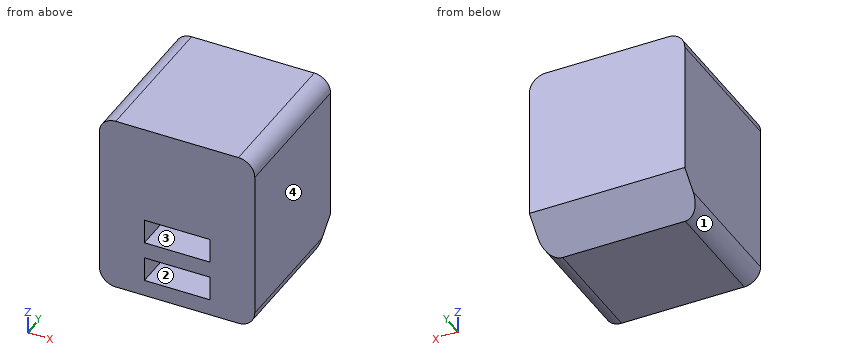
from build123d import *

# Parameters (mm, degrees)
F1_DEPTH = 28.575
F3_DEPTH = 30.1635
F6_W     = 12.7
F6_H     = 4.7625
F7_DEPTH = 12.7


with BuildPart() as f1:
    # F0 (on Front) → F1 (new body)
    with BuildSketch(Plane.XZ):
        with BuildLine():
            ThreePointArc((15.08125, 14.2875), (14.151314, 16.532564), (11.90625, 17.4625))
            Line((11.90625, 17.4625), (-11.90625, 17.4625))
            ThreePointArc((-11.90625, 17.4625), (-14.151314, 16.532564), (-15.08125, 14.2875))
            Line((-15.08125, 14.2875), (-15.08125, -14.2875))
            ThreePointArc((-15.08125, -14.2875), (-14.151314, -16.532564), (-11.90625, -17.4625))
            Line((-11.90625, -17.4625), (11.90625, -17.4625))
            ThreePointArc((11.90625, -17.4625), (14.151314, -16.532564), (15.08125, -14.2875))
            Line((15.08125, -14.2875), (15.08125, 14.2875))
        make_face()
    extrude(amount=-F1_DEPTH)

    # F2 (on face) → F3 (cut, through all)
    with BuildSketch(Plane.YZ.offset(15.08125)):
        Polygon((28.575, -17.4625), (28.575, -11.1125), (22.225, -17.4625), align=None)
    extrude(amount=-F3_DEPTH, mode=Mode.SUBTRACT)

    # F6 (on face) → F7 (cut)
    with BuildSketch(Plane.XZ):
        with Locations((0, -11.90625)):
            Rectangle(F6_W, F6_H)
        with Locations((0, -3.96875)):
            Rectangle(F6_W, F6_H)
    extrude(amount=-F7_DEPTH, mode=Mode.SUBTRACT)


solid = f1.part
Verification items for the finished model (mm, model axes). Face numbers are marked on the shaded views. Coordinates: 2 decimals unless noted, no trailing zeros. Order: outer loops, then holes, each group sorted by start corner. A loop starts at its lowest first (then second) coordinate and runs counter-clockwise, first axis right, second up.
Item 1: Section check A-A, the plane y = 9.25. Give the number of separate pieces and of enclosed holes in the cut face, then the cut area to 3 significant figures.
Filled in:
separate pieces: 1
enclosed holes: 2
area: 924 mm2
Item 2: Depth check by flat-ended pin: pin 1 (6 mm diameter, centred on x = -7, z = -12, fed in from +Y) (3 decimals); pin 2 (2.5 mm diameter, centred on x = -2, z = -11, fed in from -Y). Enter the tip coordinate at first touch or a pass-through.
Filled in:
pin 1: stops at y = 28.575
pin 2: stops at y = 12.7
Item 3: Release check for a two-part mould opening along Z. For the marked faces 1, 2, 3 and 4 record: +Z half, -Z half, draft (parallel to the pull), parting line (faces both ways), or undercut.
Filled in:
face 1: -Z half
face 2: undercut
face 3: undercut
face 4: draft
Item 4: Material ranges on L1, parallel to X at y = 4.25, z = -11; L2, parallel to Y at x = -5.5, z = -6 (3 decimals); L3, parallel to Z at x = 11.5, y = 26.5, recorded low to high.
Filled in:
L1: x = -15.08 to -6.35, 6.35 to 15.08
L2: y = 12.7 to 28.575
L3: z = -13.19 to 17.46
Item 5: Section check D-D, the plane x = 11. Enter the section's corners in (y, z) (1 decimal), then the cut area to 3 significant figures.
Filled in:
outline: (0, -17.5) - (22.2, -17.5) - (28.6, -11.1) - (28.6, 17.5) - (0, 17.5) - close
area: 978 mm2
Item 6: Section check B-B, the plane z = -3. Enter the section's corners in (x, y) (3 decimals), then the cut area to 3 significant figures.
Filled in:
outline: (-15.081, 0) - (-6.35, 0) - (-6.35, 12.7) - (6.35, 12.7) - (6.35, 0) - (15.081, 0) - (15.081, 28.575) - (-15.081, 28.575) - close
area: 701 mm2
